Verification items for the finished model (mm, model axes). A direction names the side the tool comes from. Coordinates: 2 decimals unless noted, no trailing zeros. Write each loop counter-clockwise with the first axis right and the second up, starting at its lowest first coordinate (ties: lowest second). Pieces come first, ordered by that corner, then holes. Notation, with made-up numbers: (2.25, -35.75) - (49.25, -35.75) arc R19 cw to (49.25, -1.75) - close; hole circle Ø10 at (-14, 53.5). An arc over 180 degrees is marked (long way). Use one line per item in the form item = value. Start each with the question number.
(1) Material ranges on line 1 (Y direction, x = -8.25, z = 5); line 2 (Y direction, x = 0, z = 5); line 3 (Y direction, x = -5.5, z = 5), recorded low to high. Write a range as [from, to].
(2) Tool access check on faces 5 (the cylindrical face through (-6.695, 7.709, 3.337)), 6 (the flat face through (0, 0, 0)), 7 (the flat face through (-3.5, 5, 5)), 8 (the flat face through (3.5, 5, 5)). Record the directions out of +Z, -Z, +X, -X, +Y, -Y that give a thin tool (end or side, any length) a straight path to the whole face; none if there is none.
(3) Sectioned sample at D-D (y = 5.5). Record the cut outline in (x, z), and give its area (3 significant figures).
(4) Gauge pin test, flat ends, axial feed: pin 1 Ø0.9 at (y, z) = (4, 5.5) entering from +X; pin 2 Ø1.5 at (y, z) = (5, 5) entering from -X. Record the tip position at first contact, or that the pin passes through.
(5) Sectioned sample at A-A (x = 0). Record the cut outline in (y, z).
(6) Sectioned sample at C-C (z = 9). Record the cut outline in (x, y).
(7) Sectioned sample at B-B (z = 2.25). Record the cut outline in (x, y).
(8) Mould release check, pull along X, two halves, no side actions. Record for faces 1 (the flat face through (10, 0, 5)), 2 (the flat face through (0, 10, 5)), 3 (the cylindrical face through (6.305, 7.709, 3.337)), 4 (the cylindrical face through (-0.65, 1.07, 5.07)): released by +X, released by -X, zero draft, split by the parting line, or undercut.
from build123d import *

# Parameters (mm, degrees)
SKETCH1_W           = 20
SKETCH1_H           = 20
BOSS_EXTRUDE1_DEPTH = 10
FILLET1_R           = 0.25
SKETCH2_R           = 3
CUT_EXTRUDE1_DEPTH  = 10
SKETCH3_R           = 3.5
CUT_EXTRUDE2_DEPTH  = 20
SKETCH4_R           = 1.5
CUT_EXTRUDE3_DEPTH  = 6.5
SKETCH5_R           = 1.5
CUT_EXTRUDE4_DEPTH  = 6.5
SKETCH6_R           = 1.5
CUT_EXTRUDE5_DEPTH  = 6


with BuildPart() as part:
    # Sketch1 → Boss-Extrude1 (new body)
    with BuildSketch(Plane.XY):
        Rectangle(SKETCH1_W, SKETCH1_H)
    extrude(amount=BOSS_EXTRUDE1_DEPTH)

    # Fillet1
    fillet1_edges = [part.edges().sort_by_distance(p)[0] for p in [
        (-10, 0, 10),
        (0, -10, 10),
        (10, 0, 10),
        (-10, 0, 0),
        (10, 0, 0),
        (0, 10, 10),
        (10, -10, 5),
        (-10, -10, 5),
        (-10, 10, 5),
        (10, 10, 5),
    ]]
    fillet(fillet1_edges, radius=FILLET1_R)

    # Sketch2 → Cut-Extrude1 (cut)
    with BuildSketch(Plane.XY.offset(10)):
        with Locations((0, 4)):
            Circle(SKETCH2_R)
    extrude(amount=-CUT_EXTRUDE1_DEPTH, mode=Mode.SUBTRACT)

    # Sketch3 → Cut-Extrude2 (cut)
    with BuildSketch(Plane.ZY.offset(10)):
        with Locations((5, -4.5)):
            Circle(SKETCH3_R)
    extrude(amount=-CUT_EXTRUDE2_DEPTH, mode=Mode.SUBTRACT)

    # Sketch4 → Cut-Extrude3 (cut)
    with BuildSketch(Plane.ZY.offset(10)):
        with Locations((5, 4.5)):
            Circle(SKETCH4_R)
    extrude(amount=-CUT_EXTRUDE3_DEPTH, mode=Mode.SUBTRACT)

    # Sketch5 → Cut-Extrude4 (cut)
    with BuildSketch(Plane(origin=(10, 0, 0), x_dir=(0, 0, -1), z_dir=(1, 0, 0))):
        with Locations((-5, 4.5)):
            Circle(SKETCH5_R)
    extrude(amount=-CUT_EXTRUDE4_DEPTH, mode=Mode.SUBTRACT)

    # Sketch6 → Cut-Extrude5 (cut)
    with BuildSketch(Plane(origin=(0, 10, 0), x_dir=(1, 0, 0), z_dir=(0, 1, 0))):
        with Locations((-6.5, -4.824104789)):
            Circle(SKETCH6_R)
        with Locations((6.5, -4.824104789)):
            Circle(SKETCH6_R)
    extrude(amount=-CUT_EXTRUDE5_DEPTH, mode=Mode.SUBTRACT)


solid = part.part
Answers below:
q1.line_1 = [-10, -8], [-1, 3], [6, 10]
q1.line_2 = [-10, -8], [-1, 1], [7, 10]
q1.line_3 = [-10, -8], [-1, 3]
q2.face_5 = +Y
q2.face_6 = -Z, +X, -X, +Y, -Y
q2.face_7 = -X
q2.face_8 = +X
q3.outline = (-10, 0.25) arc R0.25 ccw to (-9.75, 0) - (-2.6, 0) - (-2.6, 10) - (-9.75, 10) arc R0.25 ccw to (-10, 9.75) - (-10, 6.12) - (-7.26, 6.12) arc R1.5 cw to (-5.74, 6.12) - (-3.5, 6.12) - (-3.5, 3.88) - (-5.33, 3.88) arc R1.5 cw to (-7.67, 3.88) - (-10, 3.88) - close; (2.6, 0) - (9.75, 0) arc R0.25 ccw to (10, 0.25) - (10, 3.88) - (7.67, 3.88) arc R1.5 cw to (5.33, 3.88) - (3.5, 3.88) - (3.5, 6.12) - (5.74, 6.12) arc R1.5 cw to (7.26, 6.12) - (10, 6.12) - (10, 9.75) arc R0.25 ccw to (9.75, 10) - (2.6, 10) - close
q3.area = 117 mm2
q4.pin_1 = 3.5
q4.pin_2 = -3.5
q5.outline = (-10, 0) - (1, 0) - (1, 10) - (-9.75, 10) arc R0.25 ccw to (-10, 9.75) - close; (7, 0) - (10, 0) - (10, 9.75) arc R0.25 ccw to (9.75, 10) - (7, 10) - close; hole circle Ø7 at (-4.5, 5)
q6.outline = (-10, -9.75) arc R0.25 ccw to (-9.75, -10) - (9.75, -10) arc R0.25 ccw to (10, -9.75) - (10, 9.75) arc R0.25 ccw to (9.75, 10) - (-9.75, 10) arc R0.25 ccw to (-10, 9.75) - close; hole circle Ø6 at (0, 4)
q7.outline = (-10, -9.75) arc R0.25 ccw to (-9.75, -10) - (9.75, -10) arc R0.25 ccw to (10, -9.75) - (10, -6.67) - (-10, -6.67) - close; (-10, -2.33) - (10, -2.33) - (10, 9.75) arc R0.25 ccw to (9.75, 10) - (-9.75, 10) arc R0.25 ccw to (-10, 9.75) - close; hole circle Ø6 at (0, 4)
q8.face_1 = released by +X
q8.face_2 = zero draft
q8.face_3 = undercut
q8.face_4 = undercut
